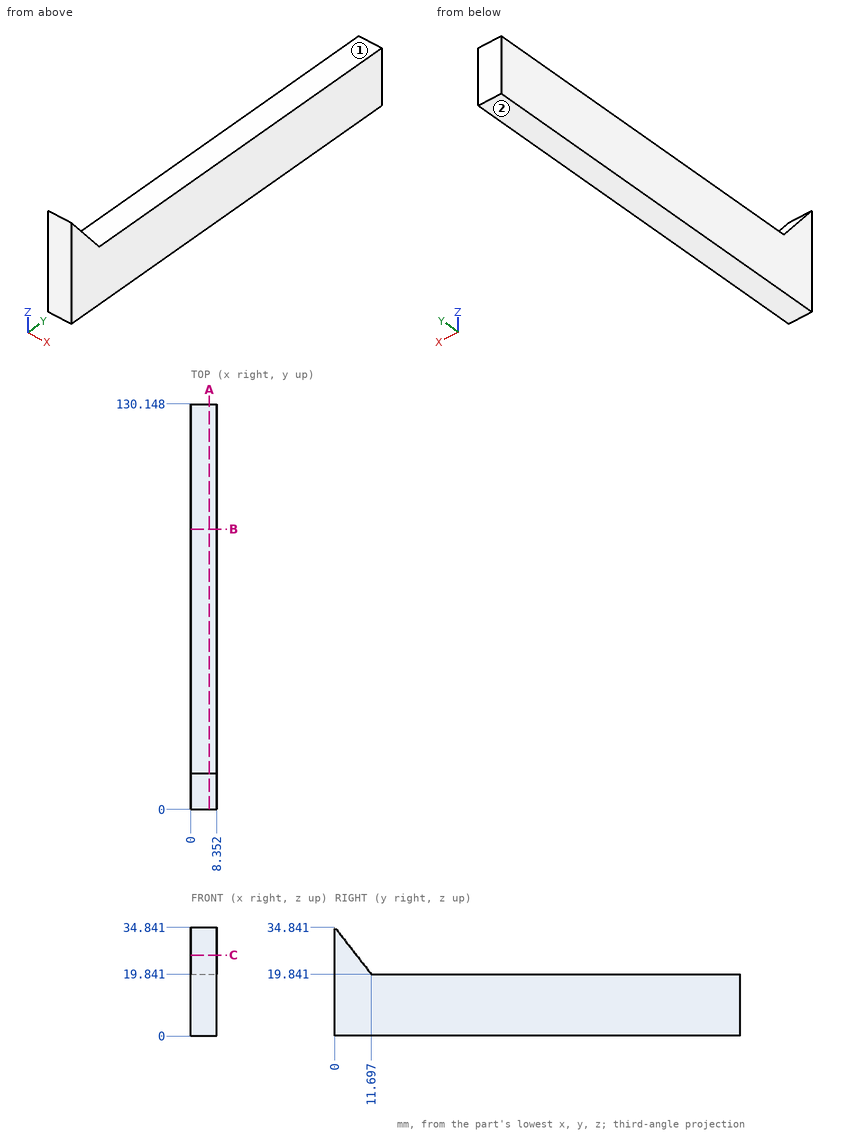
Geometry: see drawing. Coordinates: mm, zero at the bounding-box minimum. A direction names the side the tool comes from. Coordinates: 2 decimals unless noted, no trailing zeros. Loops run counter-clockwise (first coordinate to the right, second up) from the corner with the lowest first, then second, coordinate; pieces in that order, holes last. Notation, with made-up numbers: (-7, 48) - (-3, 48) arc R18 cw to (-3, 69) - close; hole circle Ø4 at (31, 80). An arc over 180 degrees is marked (long way). Return JSON: item names as keys, results as strings.
Q1. Contact query for flat-ended pins moving along their axis: P1, Ø4, axis at x = 3.5, y = 60.5, coming from the +Z side; P2, Ø2, axis at x = 5.5, z = 27.5, coming from the +Y side (1 decimal). Output: stop coordinate, or through.
Results:
{"P1": "z = 19.84", "P2": "y = 6.5"}
Q2. Section C-C, the plane z = 26. Return loops of the section in (x, y).
Results:
{"outline": "(0, 0) - (8.35, 0) - (8.35, 6.89) - (0, 6.89) - close"}
Q3. Access query for the marked faces 1 and 2. Directions: +Z, -Z, +X, -X, +Y, -Y. A direction counts if a zero-diameter tool reaches every point of the face in a straight line with its end or side. Return the directions, or none.
Results:
{"face 1": "+Z, +X, -X, +Y", "face 2": "-Z, +X, -X, +Y, -Y"}
Q4. Material intervals for line 1 along Z through (x, y) = (7.75, 49); line 2 along Y through (x, z) = (0.5, 27) (1 decimal); line 3 along Y through (x, z) = (0.75, 20.5), sorted ascending.
Results:
{"line 1": "0 to 19.84", "line 2": "0 to 6.1", "line 3": "0 to 11.18"}
Q5. Section B-B, the plane y = 90. Return loops of the section in (x, z), plus the area to 3 significant figures.
Results:
{"outline": "(0, 0) - (8.35, 0) - (8.35, 19.84) - (0, 19.84) - close", "area": "166 mm2"}
Q6. Section A-A, the plane x = 6. Return loops of the section in (y, z).
Results:
{"outline": "(0, 0) - (130.15, 0) - (130.15, 19.84) - (11.7, 19.84) - (0, 34.84) - close"}
